Check sheet for the drawn part. Datum: minimum x, y, z corner. Units: mm. Coordinates: 2 decimals unless noted, no trailing zeros. Loops run counter-clockwise (first coordinate to the right, second up) from the corner with the lowest first, then second, coordinate; pieces in that order, holes last.
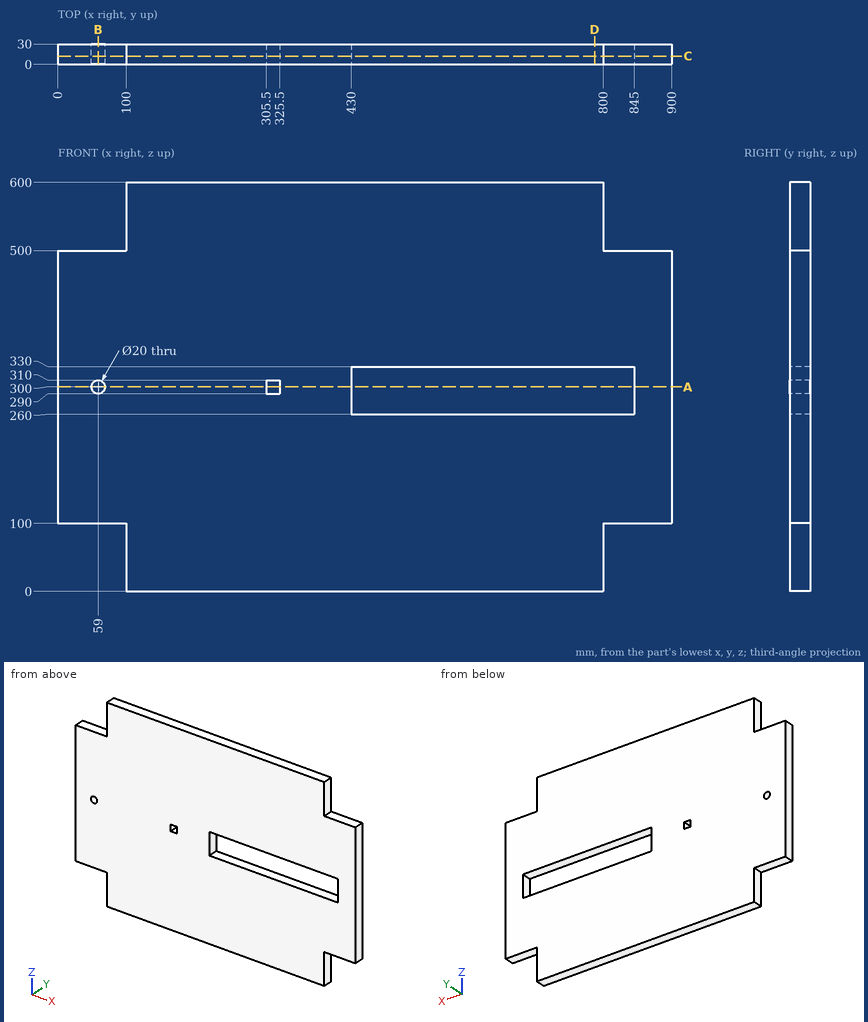
(1) Sectioned sample at D-D on x = 787. Record the cut outline in (y, z), and give its area (3 significant figures).
Findings:
outline: (0, 0) - (30, 0) - (30, 260) - (0, 260) - close; (0, 330) - (30, 330) - (30, 600) - (0, 600) - close
area: 15,900 mm2
(2) Scan lines: L1, parallel to X at y = 20.5, z = 300; L2, parallel to X at y = 20.25, z = 275; L3, parallel to Z at x = 680, y = 27. Record each from-to range of solid material in increasing order.
Findings:
L1: x = 0 to 49, 69 to 305.5, 325.5 to 430, 845 to 900
L2: x = 0 to 430, 845 to 900
L3: z = 0 to 260, 330 to 600
(3) Sectioned sample at A-A on z = 300. Record the cut outline in (x, y), and give its area (4 significant figures).
Findings:
outline: (0, 0) - (49, 0) - (49, 30) - (0, 30) - close; (69, 0) - (305.5, 0) - (305.5, 30) - (69, 30) - close; (325.5, 0) - (430, 0) - (430, 30) - (325.5, 30) - close; (845, 0) - (900, 0) - (900, 30) - (845, 30) - close
area: 13,350 mm2
(4) Sectioned sample at B-B on x = 59. Record the cut outline in (y, z).
Findings:
outline: (0, 100) - (30, 100) - (30, 290) - (0, 290) - close; (0, 310) - (30, 310) - (30, 500) - (0, 500) - close
(5) Sectioned sample at C-C on y = 12.25. Record the cut outline in (x, z), and give its area (3 significant figures).
Findings:
outline: (0, 100) - (100, 100) - (100, 0) - (800, 0) - (800, 100) - (900, 100) - (900, 500) - (800, 500) - (800, 600) - (100, 600) - (100, 500) - (0, 500) - close; hole circle Ø20 at (59, 300); hole (305.5, 290) - (325.5, 290) - (325.5, 310) - (305.5, 310) - close; hole (430, 260) - (845, 260) - (845, 330) - (430, 330) - close
area: 470,000 mm2
(6) Gauge pin test, flat ends, axial feed: pin 1 Ø9 at (x, y) = (52.5, 11) entering from -Z; pin 2 Ø16 at (y, z) = (11, 302) entering from -X; pin 3 Ø3 at (y, z) = (25.5, 90.5) entering from -X; pin 4 Ø15 at (y, z) = (9, 567) entering from +X. Record the tip position at first contact, or that the pin passes through.
Findings:
pin 1: stops at z = 100
pin 2: stops at x = 0
pin 3: stops at x = 100
pin 4: stops at x = 800
